from build123d import *

# Parameters (mm, degrees)
EXTRUDE_1_DEPTH = 3
SKETCH_2_R      = 9.5
EXTRUDE_2_DEPTH = 13.6
SKETCH_3_R      = 5.8
EXTRUDE_3_DEPTH = 1.3


with BuildPart() as part:
    # 草图1 → 凸台-拉伸1 (new body)
    with BuildSketch(Plane(origin=(0, 0, 0), x_dir=(1, 0, 0), z_dir=(0, 1, 0))):
        Polygon((0, 12.6), (-10.911920088, 6.3), (-10.911920088, -6.3), (0, -12.6), (10.911920088, -6.3), (10.911920088, 6.3), align=None)
    extrude(amount=EXTRUDE_1_DEPTH)

    # 草图2 → 凸台-拉伸2 (add)
    with BuildSketch(Plane.XZ):
        with Locations(Location((0, 0, 0), (0, 0, 270))):
            Circle(SKETCH_2_R)
    extrude(amount=EXTRUDE_2_DEPTH)

    # 草图3 → 凸台-拉伸3 (add)
    with BuildSketch(Plane(origin=(0, 3, 0), x_dir=(1, 0, 0), z_dir=(0, 1, 0))):
        with Locations(Location((0, 0, 0), (0, 0, 270))):
            Circle(SKETCH_3_R)
    extrude(amount=EXTRUDE_3_DEPTH)


solid = part.part
Design review of the part built by this model. Coordinates are the model's own, in mm. A direction names the side the tool comes from. Coordinates: 2 decimals unless noted, no trailing zeros. Loops run counter-clockwise (first coordinate to the right, second up) from the corner with the lowest first, then second, coordinate; pieces in that order, holes last.
Item 1: Wall thickness on L1, parallel to Y at x = 9.75, z = -6; L2, parallel to Y at x = -0.5, z = 9; L3, parallel to Z at x = 0.25, y = -3.25: over which ranges is each line inside the solid? List them lowest first.
Completed:
L1: y = 0 to 3
L2: y = -13.6 to 3
L3: z = -9.5 to 9.5
Item 2: For faces 1 (the flat face through (-3.3, 0, 9.3)), 2 (the flat face through (10.912, 1, 0)), 3 (the flat face through (-2.6, 3, 5.4)), list the 3-axis set-ups (+Z, -Z, +X, -X, +Y, -Y) from which the entire face can be reached by the end or side of a thin tool; tool diameter is ignored.
Completed:
face 1: -Y
face 2: +Z, -Z, +X, +Y, -Y
face 3: +Y
Item 3: Add section A-A (z = 0). Write out the cut boundary in (x, y).
Completed:
outline: (-10.91, 0) - (-9.5, 0) - (-9.5, -13.6) - (9.5, -13.6) - (9.5, 0) - (10.91, 0) - (10.91, 3) - (5.8, 3) - (5.8, 4.3) - (-5.8, 4.3) - (-5.8, 3) - (-10.91, 3) - close
Item 4: Add section C-C (y = -11.5). Write out the cut boundary in (x, z), and give its area (3 significant figures).
Completed:
outline: circle Ø19 at (0, 0)
area: 284 mm2
Item 5: Add section B-B (x = 4.25). Write out the cut boundary in (y, z).
Completed:
outline: (-13.6, -8.5) - (0, -8.5) - (0, -10.15) - (3, -10.15) - (3, -3.95) - (4.3, -3.95) - (4.3, 3.95) - (3, 3.95) - (3, 10.15) - (0, 10.15) - (0, 8.5) - (-13.6, 8.5) - close
Item 6: Clearance check with flat-ended pins moving along their axes: pin 1 (1.5 mm diameter, centred on x = 4.5, y = 0.5, fed in from +Z); pin 2 (12 mm diameter, centred on x = 3, z = 9.5, fed in from -Y); pin 3 (1.5 mm diameter, centred on x = -1.5, y = 1.5, fed in from +Z); pin 4 (8 mm diameter, centred on x = -8, y = -7, fed in from -Z). State where each tip first meets the part, or that it passes through.
Completed:
pin 1: stops at z = 10.43
pin 2: stops at y = -13.6
pin 3: stops at z = 12.17
pin 4: stops at z = -8.62
Item 7: Add section D-D (x = 9). Write out the cut boundary in (y, z), and give its area (3 significant figures).
Completed:
outline: (-13.6, -3.04) - (0, -3.04) - (0, -7.4) - (3, -7.4) - (3, 7.4) - (0, 7.4) - (0, 3.04) - (-13.6, 3.04) - close
area: 127 mm2
